from build123d import *

# Parameters (mm, degrees)
SKETCH1_W                    = 100
SKETCH1_H                    = 20
SKETCH1_R                    = 1.6
EXTRUDE_BASE_DEPTH           = 5
SKETCH2_W                    = 100
SKETCH2_H                    = 5
EXTRUDE_VERTICAL_CLAMP_DEPTH = 20
SKETCH3_W                    = 100
SKETCH3_H                    = 5
EXTRUDE_CLAMP_ROOF_DEPTH     = 7
SKETCH5_W                    = 100
SKETCH5_H                    = 10
SKETCH5_R                    = 1.6
BOSS_EXTRUDE4_DEPTH          = 5
SKETCH4_R                    = 3.75
CUT_EXTRUDE1_DEPTH           = 2.5


with BuildPart() as part:
    # Sketch1 → Extrude-Base (new body)
    with BuildSketch(Plane(origin=(0, 0, 0), x_dir=(1, 0, 0), z_dir=(0, 1, 0))):
        with Locations((50, 10)):
            Rectangle(SKETCH1_W, SKETCH1_H)
        with Locations(Location((35, 7, 0), (0, 0, 270))):
            Circle(SKETCH1_R, mode=Mode.SUBTRACT)
        with Locations(Location((65, 7, 0), (0, 0, 270))):
            Circle(SKETCH1_R, mode=Mode.SUBTRACT)
    extrude(amount=EXTRUDE_BASE_DEPTH)

    # Sketch2 → Extrude-Vertical clamp (add)
    with BuildSketch(Plane(origin=(0, 5, 0), x_dir=(1, 0, 0), z_dir=(0, 1, 0))):
        with Locations((50, 17.5)):
            Rectangle(SKETCH2_W, SKETCH2_H)
    extrude(amount=EXTRUDE_VERTICAL_CLAMP_DEPTH)

    # Sketch3 → Extrude-Clamp Roof (add)
    with BuildSketch(Plane.XY.offset(-15)):
        with Locations((50, 22.5)):
            Rectangle(SKETCH3_W, SKETCH3_H)
    extrude(amount=EXTRUDE_CLAMP_ROOF_DEPTH)

    # Sketch5 → Boss-Extrude4 (add)
    with BuildSketch(Plane(origin=(0, 0, 0), x_dir=(1, 0, 0), z_dir=(0, 1, 0))):
        with Locations((50, 25)):
            Rectangle(SKETCH5_W, SKETCH5_H)
        with Locations(Location((70, 25, 0), (0, 0, 270))):
            Circle(SKETCH5_R, mode=Mode.SUBTRACT)
        with Locations(Location((30, 25, 0), (0, 0, 270))):
            Circle(SKETCH5_R, mode=Mode.SUBTRACT)
    extrude(amount=BOSS_EXTRUDE4_DEPTH)

    # Sketch4 → Cut-Extrude1 (cut)
    with BuildSketch(Plane(origin=(0, 5, 0), x_dir=(1, 0, 0), z_dir=(0, 1, 0))):
        with Locations(Location((35, 7, 0), (0, 0, 270))):
            Circle(SKETCH4_R)
        with Locations(Location((65, 7, 0), (0, 0, 270))):
            Circle(SKETCH4_R)
        with Locations(Location((30, 25, 0), (0, 0, 270))):
            Circle(SKETCH4_R)
        with Locations(Location((70, 25, 0), (0, 0, 270))):
            Circle(SKETCH4_R)
    extrude(amount=-CUT_EXTRUDE1_DEPTH, mode=Mode.SUBTRACT)


solid = part.part
Build history of the part. All positions in model axes, mm. A direction names the side the tool comes from. Coordinates: 2 decimals unless noted, no trailing zeros. Write each loop counter-clockwise with the first axis right and the second up, starting at its lowest first coordinate (ties: lowest second). Pieces come first, ordered by that corner, then holes.
(1) Mould opens along Z. For faces 1 (the cylindrical face through (66.586, 1.232, -7.208)), 2 (the flat face through (49, 2, -30)), 3 (the flat face through (49, 23, -8)) say: pulls with the +Z half, pulls with the -Z half, needs draft (parallel to the pull), parting line crosses it, or undercut.
(2) Cut at D-D on x = 30. List the corners of the cut face in (y, z).
(3) Drill centre lines: line 1 (X direction, y = 1.9, z = -7); line 2 (Y direction, x = 57, z = -8.5); line 3 (Z direction, x = 70, y = 0.7). Where is each one in solid material? Low to high.
(4) Cut at B-B on x = 45. List the corners of the cut face in (y, z).
(5) Cut at A-A on z = -11.75. List the corners of the cut face in (x, y).
(6) Cut at C-C on z = -25. List the corners of the cut face in (x, y).
(7) Pin check, flat tips, straight feed: pin 1 Ø10 at (x, y) = (74, 18) entering from +Z; pin 2 Ø8 at (y, z) = (12, -10.5) entering from +X; pin 3 Ø3 at (x, z) = (76.5, -26) entering from +Y; pin 4 Ø3 at (x, z) = (35, -7) entering from -Y. Stop position of each tip, or through.
(8) 3-axis set-ups, long thin cutter, end or side, ignore diameter. For faces 4 (the flat face through (35, 2.5, -5)), 5 (the flat face through (28, 2.5, -25)), 6 (the flat face through (49, 2, 0)), 7 (the flat face through (49, 20, -12)), 8 (the flat face through (49, 15, -20)): which of +Z, -Z, +X, -X, +Y, -Y reach the whole face in a straight line?
Working result:
1. face 1: undercut
1. face 2: pulls with the -Z half
1. face 3: pulls with the +Z half
2. outline: (0, -30) - (5, -30) - (5, -28.75) - (2.5, -28.75) - (2.5, -26.6) - (0, -26.6) - close; (0, -23.4) - (2.5, -23.4) - (2.5, -21.25) - (5, -21.25) - (5, -20) - (25, -20) - (25, -8) - (20, -8) - (20, -15) - (5, -15) - (5, 0) - (0, 0) - close
3. line 1: x = 0 to 33.4, 36.6 to 63.4, 66.6 to 100
3. line 2: y = 0 to 5, 20 to 25
3. line 3: z = -30 to -26.6, -23.4 to 0
4. outline: (0, -30) - (5, -30) - (5, -20) - (25, -20) - (25, -8) - (20, -8) - (20, -15) - (5, -15) - (5, 0) - (0, 0) - close
5. outline: (0, 0) - (100, 0) - (100, 5) - (0, 5) - close; (0, 20) - (100, 20) - (100, 25) - (0, 25) - close
6. outline: (0, 0) - (28.4, 0) - (28.4, 2.5) - (26.25, 2.5) - (26.25, 5) - (0, 5) - close; (31.6, 0) - (68.4, 0) - (68.4, 2.5) - (66.25, 2.5) - (66.25, 5) - (33.75, 5) - (33.75, 2.5) - (31.6, 2.5) - close; (71.6, 0) - (100, 0) - (100, 5) - (73.75, 5) - (73.75, 2.5) - (71.6, 2.5) - close
7. pin 1: stops at z = -8
7. pin 2: passes through
7. pin 3: stops at y = 5
7. pin 4: stops at y = 20
8. face 4: none
8. face 5: +Y
8. face 6: +Z, +X, -X, +Y, -Y
8. face 7: +Z, +X, -X
8. face 8: -Z, +X, -X, +Y
